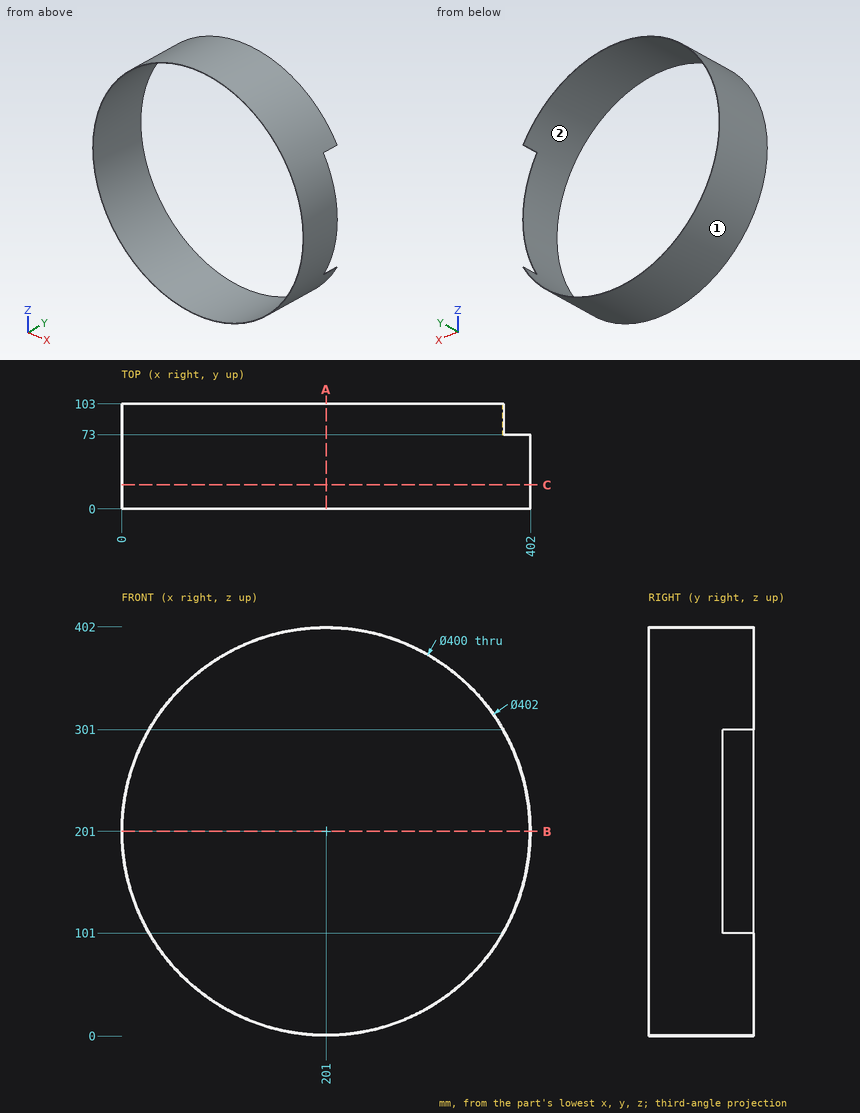
Print and shaded views of the part. All mm, measured from the part's lowest x, y and z. Coordinates: 2 decimals unless noted, no trailing zeros. Write each loop counter-clockwise with the first axis right and the second up, starting at its lowest first coordinate (ties: lowest second). Pieces come first, ordered by that corner, then holes. Notation, with made-up numbers: (7.5, 84) -> (17.5, 84) arc R26 ccw to (17.5, 110) -> close; hole circle Ø6 at (85.5, 34.5). An arc over 180 degrees is marked (long way). Use CSV: the item, a comma, the result in double quotes. Start each with the question number.
Q1. Cut at A-A, the plane x = 201. List the corners of the cut face in (y, z), then the cut area to 3 significant figures.
Q2. Drill centre lines: probe 1 along Z at (x, y) = (195.5, 56); probe 2 along Z at (x, y) = (201, 53). Where is each one in solid material? Low to high.
Q3. Cut at B-B, the plane z = 201. List the corners of the cut face in (x, y), then the cut area to 3 significant figures.
Q4. Cut at C-C, the plane y = 23.5. List the corners of the cut face in (x, z).
Q5. Pull direction Z, two halves, no side cores. Call the marked faces 1 and 2: released by +Z, released by -Z, zero draft, split by the parting line, or undercut.
Q6. Flat gauge pins, fed straight in: pin 1 Ø22 at (x, z) = (392.5, 188) entering from +Y; pin 2 Ø3 at (x, y) = (264.5, 29.5) entering from -Z; pin 3 Ø1.5 at (x, y) = (322, 61) entering from +Z. Where does each tip first touch, or does it go through?
Checked values:
1,outline,"(0, 0) -> (103, 0) -> (103, 1) -> (0, 1) -> close; (0, 401) -> (103, 401) -> (103, 402) -> (0, 402) -> close"
1,area,"206 mm²"
2,probe 1,"z = 0.08 to 1.08, 400.92 to 401.92"
2,probe 2,"z = 0 to 1, 401 to 402"
3,outline,"(0, 0) -> (1, 0) -> (1, 103) -> (0, 103) -> close; (401, 0) -> (402, 0) -> (402, 73) -> (401, 73) -> close"
3,area,"176 mm²"
4,outline,"circle Ø402 at (201, 201); hole circle Ø400 at (201, 201)"
5,face 1,"split by the parting line"
5,face 2,"undercut"
6,pin 1,"stops at y = 73"
6,pin 2,"stops at z = 9.8"
6,pin 3,"stops at z = 362.06"
